Part print with two shaded views. Sizes in mm from the minimum x, y, z corner. A direction names the side the tool comes from. Give positions to 0.01 mm unless a question says otherwise; leave off trailing zeros. Write each loop counter-clockwise with the first axis right and the second up, starting at its lowest first coordinate (ties: lowest second). Pieces come first, ordered by that corner, then holes. Notation, with made-up numbers: (-33, 43) -> (14, 43) arc R30 ccw to (14, 76) -> close; hole circle Ø6 at (-30.75, 43). An arc over 180 degrees is marked (long way). Answer as a JSON object with one key per item and string values.
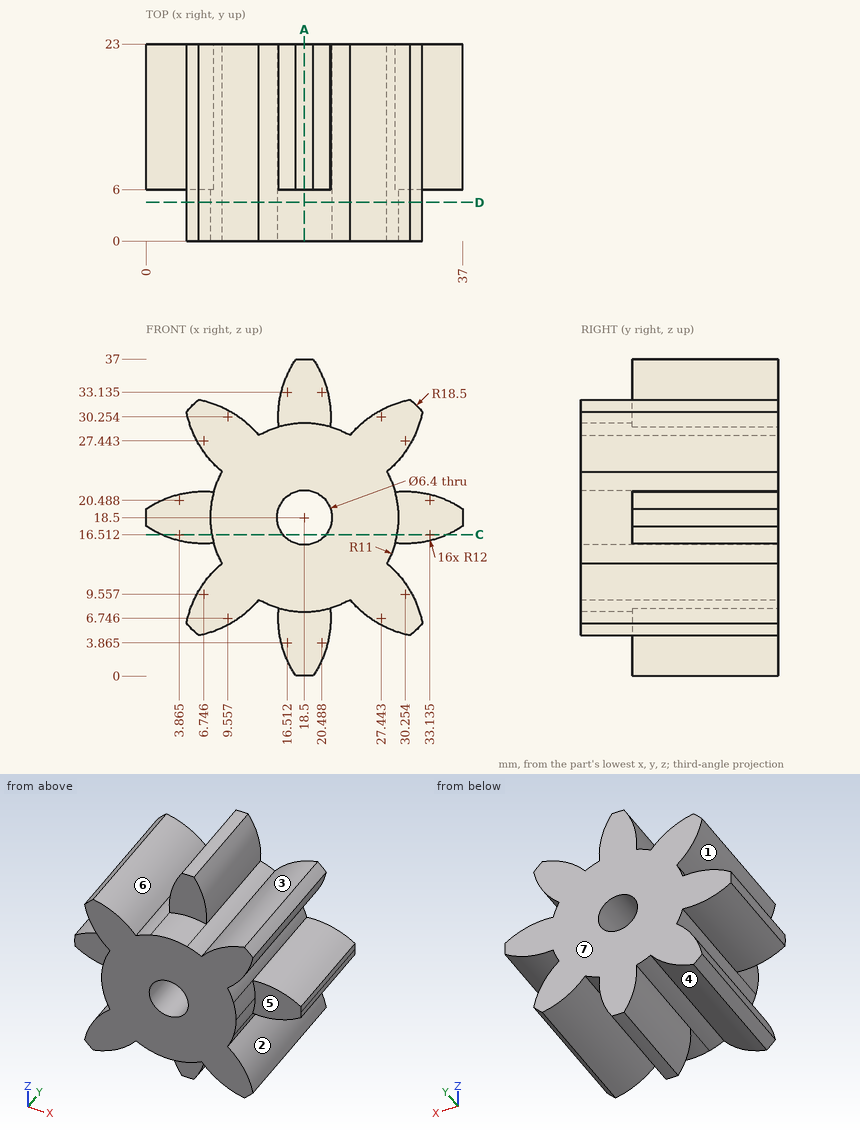
1) Slice it at A-A (x = 18.5). List the corners of the cut face in (y, z), then the cut area to 3 significant figures.
Model answer:
{"outline": "(0, 7.5) -> (6, 7.5) -> (6, 0) -> (23, 0) -> (23, 15.3) -> (0, 15.3) -> close; (0, 21.7) -> (23, 21.7) -> (23, 37) -> (6, 37) -> (6, 29.5) -> (0, 29.5) -> close", "area": "614 mm2"}
2) 3-axis set-ups, long thin cutter, end or side, ignore diameter. For the marked faces 1, 2, 3 and 4: which of +Z, -Z, +X, -X, +Y, -Y reach the whole face in a straight line?
Model answer:
{"face 1": "-X, +Y, -Y", "face 2": "+X, +Y, -Y", "face 3": "+Z, +Y, -Y", "face 4": "-Z, +Y, -Y"}
3) Mould opens along Z. For the marked faces 5, 6 and 7 say: released by +Z, released by -Z, zero draft, split by the parting line, or undercut.
Model answer:
{"face 5": "undercut", "face 6": "released by +Z", "face 7": "zero draft"}
4) Wall check: probe 1 along X at (y, z) = (10, 18.5); probe 2 along Y at (x, z) = (31.5, 16); probe 3 along Z at (x, y) = (31.5, 10) (1 decimal). Give the ranges that are in metal, low to high.
Model answer:
{"probe 1": "x = 0 to 15.3, 21.7 to 37", "probe 2": "y = 6 to 23", "probe 3": "z = 5.3 to 8.6, 15.5 to 21.5, 28.4 to 31.7"}
5) Slice it at D-D (y = 4.5). List the corners of the cut face in (x, z) (1 decimal), then the cut area to 3 significant figures.
Model answer:
{"outline": "(4.7, 6.1) arc R18.5 ccw to (6.1, 4.7) arc R12 ccw to (13.1, 8.9) arc R11 ccw to (23.9, 8.9) arc R12 ccw to (30.9, 4.7) arc R18.5 ccw to (32.3, 6.1) arc R12 ccw to (28.1, 13.1) arc R11 ccw to (28.1, 23.9) arc R12 ccw to (32.3, 30.9) arc R18.5 ccw to (30.9, 32.3) arc R12 ccw to (23.9, 28.1) arc R11 ccw to (13.1, 28.1) arc R12 ccw to (6.1, 32.3) arc R18.5 ccw to (4.7, 30.9) arc R12 ccw to (8.9, 23.9) arc R11 ccw to (8.9, 13.1) arc R12 ccw to start; hole circle Ø6.4 at (18.5, 18.5)", "area": "499 mm2"}
6) Slice it at C-C (z = 16.5). List the corners of the cut face in (x, y), then the cut area to 3 significant figures.
Model answer:
{"outline": "(1.82, 6) -> (7.68, 6) -> (7.68, 0) -> (16, 0) -> (16, 23) -> (1.82, 23) -> close; (21, 0) -> (29.32, 0) -> (29.32, 6) -> (35.18, 6) -> (35.18, 23) -> (21, 23) -> close", "area": "582 mm2"}
7) Pin check, flat tips, straight feed: pin 1 (5 mm diameter, centred on x = 34, z = 17.5, fed in from -Y); pin 2 (8 mm diameter, centred on x = 30, y = 17, fed in from -Z); pin 3 (6 mm diameter, centred on y = 5, z = 23, fed in from +X); pin 4 (1.5 mm diameter, centred on x = 22.5, z = 5.5, fed in from -Y). Stop position of each tip, or through.
Model answer:
{"pin 1": "stops at y = 6", "pin 2": "stops at z = 4.73", "pin 3": "stops at x = 35.85", "pin 4": "passes through"}
